Part print with two shaded views. Sizes in mm from the minimum x, y, z corner. A direction names the side the tool comes from. Coordinates: 2 decimals unless noted, no trailing zeros. Write each loop counter-clockwise with the first axis right and the second up, starting at its lowest first coordinate (ties: lowest second). Pieces come first, ordered by that corner, then holes. Notation, with made-up numbers: (25.5, 22.25) - (75.5, 22.25) arc R25 cw to (75.5, 55.25) - close; hole circle Ø9 at (31, 69.25). An arc over 180 degrees is marked (long way). Answer in a Markdown table with one row per item. Add a question column.
Q1. Band-saw the part on A-A (x = 20). List the corners of the cut face in (y, z) (1 decimal), and give its area (3 significant figures).
Q2. Two-plate mould, pull along Y, no slides. Class the marked faces 4, 5 and 6: +Y half, -Y half, draft (parallel to the pull), parting line (faces both ways), or undercut.
Q3. Band-saw the part on D-D (z = 38). List the corners of the cut face in (x, y) (1 decimal).
Q4. 3-axis set-ups, long thin cutter, end or side, ignore diameter. For the marked faces 1, 2 and 3: which of +Z, -Z, +X, -X, +Y, -Y reach the whole face in a straight line?
Q5. Drill centre lines: line 1 along Y through (x, z) = (42, 26); line 2 along Z through (x, y) = (27.5, 3.5); line 3 along Y through (x, z) = (8, 30). Where is each one in solid material? Low to high. Write a range as from..to.
Q6. Band-saw the part on C-C (z = 28). List the corners of the cut face in (x, y) (1 decimal).
Q7. Band-saw the part on B-B (x = 32). List the corners of the cut face in (y, z).
Q8. Pin check, flat tips, straight feed: pin 1 (4.5 mm diameter, centred on x = 23.5, y = 21, fed in from +Z); pin 2 (9 mm diameter, centred on x = 20, y = 20, fed in from +Z); pin 3 (11 mm diameter, centred on x = 23.5, z = 23, fed in from -Y). Stop position of each tip, or through.
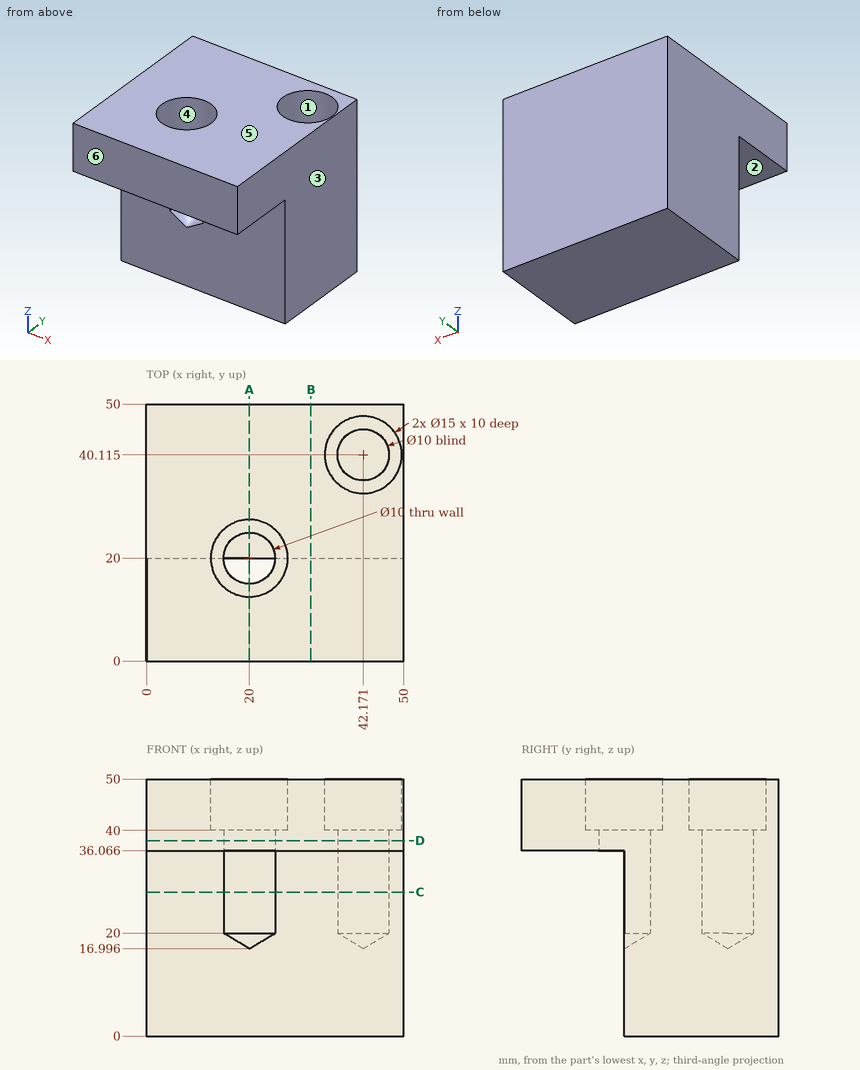
Checked values:
| question | item | result |
|---|---|---|
| 1 | outline | (0, 36.1) - (15, 36.1) - (15, 40) - (12.5, 40) - (12.5, 50) - (0, 50) - close; (20, 0) - (50, 0) - (50, 50) - (27.5, 50) - (27.5, 40) - (25, 40) - (25, 20) - (20, 17) - close |
| 1 | area | 1,500 mm² |
| 2 | face 4 | undercut |
| 2 | face 5 | draft |
| 2 | face 6 | -Y half |
| 3 | outline | (0, 0) - (50, 0) - (50, 50) - (0, 50) - close; hole circle Ø10 at (20, 20); hole circle Ø10 at (42.2, 40.1) |
| 4 | face 1 | +Z |
| 4 | face 2 | -Z, +X, -X, -Y |
| 4 | face 3 | +Z, -Z, +X, +Y, -Y |
| 5 | line 1 | y = 20..35.12, 45.11..50 |
| 5 | line 2 | z = 36.07..50 |
| 5 | line 3 | y = 20..50 |
| 6 | outline | (0, 20) - (15, 20) arc R5 cw to (25, 20) - (50, 20) - (50, 50) - (0, 50) - close; hole circle Ø10 at (42.2, 40.1) |
| 7 | outline | (0, 36.07) - (20, 36.07) - (20, 0) - (50, 0) - (50, 50) - (0, 50) - close |
| 8 | pin 1 | stops at z = 40 |
| 8 | pin 2 | stops at z = 19.7 |
| 8 | pin 3 | stops at y = 20 |
